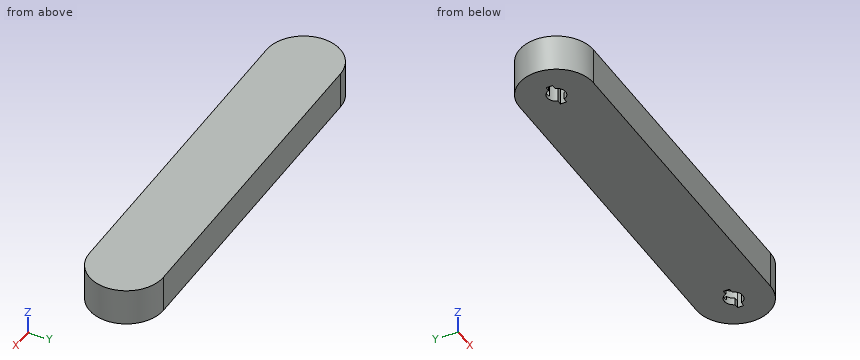
from build123d import *

# Parameters (mm, degrees)
BOSS_EXTRUDE1_DEPTH = 12.7
CUT_EXTRUDE1_DEPTH  = 6.35
CUT_EXTRUDE4_START  = 3.81
CUT_EXTRUDE4_DEPTH  = 3.81
CUT_EXTRUDE5_START  = 5.08
CUT_EXTRUDE5_DEPTH  = 5.08


with BuildPart() as part:
    # Sketch1 → Boss-Extrude1 (new body)
    with BuildSketch(Plane.XY):
        with BuildLine():
            Line((0, 0), (114.3, 0))
            ThreePointArc((114.3, 0), (127, -12.7), (114.3, -25.4))
            Line((114.3, -25.4), (0, -25.4))
            ThreePointArc((0, -25.4), (-12.7, -12.7), (0, 0))
        make_face()
    extrude(amount=-BOSS_EXTRUDE1_DEPTH)

    # Sketch2 → Cut-Extrude1 (cut)
    with BuildSketch(Plane(origin=(0, 0, -12.7), x_dir=(-1, 0, 0), z_dir=(0, 0, -1))):
        with BuildLine():
            Line((-118.872586333, -11.6205), (-118.872586333, -13.7795))
            Line((-118.872586333, -13.7795), (-117.285850758, -13.7795))
            ThreePointArc((-117.285850758, -13.7795), (-114.3, -15.875), (-111.314149242, -13.7795))
            Line((-111.314149242, -13.7795), (-109.727413667, -13.7795))
            Line((-109.727413667, -13.7795), (-109.727413667, -11.6205))
            Line((-109.727413667, -11.6205), (-111.314149242, -11.6205))
            ThreePointArc((-111.314149242, -11.6205), (-114.3, -9.525), (-117.285850758, -11.6205))
            Line((-117.285850758, -11.6205), (-118.872586333, -11.6205))
        make_face()
        with BuildLine():
            Line((-4.572586333, -11.6205), (-2.985850758, -11.6205))
            ThreePointArc((-2.985850758, -11.6205), (0, -9.525), (2.985850758, -11.6205))
            Line((2.985850758, -11.6205), (4.572586333, -11.6205))
            Line((4.572586333, -11.6205), (4.572586333, -13.7795))
            Line((4.572586333, -13.7795), (2.985850758, -13.7795))
            ThreePointArc((2.985850758, -13.7795), (0, -15.875), (-2.985850758, -13.7795))
            Line((-2.985850758, -13.7795), (-4.572586333, -13.7795))
            Line((-4.572586333, -13.7795), (-4.572586333, -11.6205))
        make_face()
    extrude(amount=-CUT_EXTRUDE1_DEPTH, mode=Mode.SUBTRACT)

    # Sketch3 → Cut-Extrude4 (cut)
    with BuildSketch(Plane(origin=(0, 0, -6.35), x_dir=(-1, 0, 0), z_dir=(0, 0, -1)).offset(CUT_EXTRUDE4_START)):
        with BuildLine():
            ThreePointArc((-113.2205, -8.127413667), (-116.769985033, -8.703371426), (-118.872586333, -11.6205))
            Line((-118.872586333, -11.6205), (-117.285850758, -11.6205))
            ThreePointArc((-117.285850758, -11.6205), (-115.647993548, -9.825362911), (-113.2205, -9.714149242))
            Line((-113.2205, -9.714149242), (-113.2205, -8.127413667))
        make_face()
        with BuildLine():
            Line((-109.727413667, -13.7795), (-111.314149242, -13.7795))
            ThreePointArc((-111.314149242, -13.7795), (-112.952006452, -15.574637089), (-115.3795, -15.685850758))
            Line((-115.3795, -15.685850758), (-115.3795, -17.272586333))
            ThreePointArc((-115.3795, -17.272586333), (-111.830014967, -16.696628574), (-109.727413667, -13.7795))
        make_face()
        with BuildLine():
            ThreePointArc((-1.0795, -8.127413667), (2.469985033, -8.703371426), (4.572586333, -11.6205))
            Line((4.572586333, -11.6205), (2.985850758, -11.6205))
            ThreePointArc((2.985850758, -11.6205), (1.347993548, -9.825362911), (-1.0795, -9.714149242))
            Line((-1.0795, -9.714149242), (-1.0795, -8.127413667))
        make_face()
        with BuildLine():
            ThreePointArc((1.0795, -17.272586333), (-2.469985033, -16.696628574), (-4.572586333, -13.7795))
            Line((-4.572586333, -13.7795), (-2.985850758, -13.7795))
            ThreePointArc((-2.985850758, -13.7795), (-1.347993548, -15.574637089), (1.0795, -15.685850758))
            Line((1.0795, -15.685850758), (1.0795, -17.272586333))
        make_face()
    extrude(amount=-CUT_EXTRUDE4_DEPTH, mode=Mode.SUBTRACT)

    # Sketch4 → Cut-Extrude5 (cut)
    with BuildSketch(Plane(origin=(0, 0, -6.35), x_dir=(-1, 0, 0), z_dir=(0, 0, -1)).offset(CUT_EXTRUDE5_START)):
        with BuildLine():
            Line((-113.2205, -9.714149242), (-113.2205, -8.127413667))
            Line((-113.2205, -8.127413667), (-115.3795, -8.127413667))
            Line((-115.3795, -8.127413667), (-115.3795, -9.714149242))
            ThreePointArc((-115.3795, -9.714149242), (-115.099019405, -9.627184843), (-114.8117038, -9.566506068))
            ThreePointArc((-114.8117038, -9.566506068), (-114.006661019, -9.538579869), (-113.2205, -9.714149242))
        make_face()
        with BuildLine():
            ThreePointArc((-115.3795, -15.685850758), (-114.3, -15.875), (-113.2205, -15.685850758))
            Line((-113.2205, -15.685850758), (-113.2205, -17.272586333))
            Line((-113.2205, -17.272586333), (-115.3795, -17.272586333))
            Line((-115.3795, -17.272586333), (-115.3795, -15.685850758))
        make_face()
    cut_extrude5 = extrude(amount=-CUT_EXTRUDE5_DEPTH, mode=Mode.SUBTRACT)

    # Mirror2: Cut-Extrude5 across plane
    add(cut_extrude5.mirror(Plane(origin=(57.15, 0, 0), x_dir=(0, 0, 1), z_dir=(1, 0, 0))), mode=Mode.SUBTRACT)


solid = part.part
Check sheet for the modelled part. Datum: model origin and axes. Units: mm. Coordinates: 2 decimals unless noted, no trailing zeros. Write each loop counter-clockwise with the first axis right and the second up, starting at its lowest first coordinate (ties: lowest second). Pieces come first, ordered by that corner, then holes.
Item 1: Cross-section at B-B on z = -1.75. Record the boundary of the cut face in (x, y).
Numbers:
outline: (0, -25.4) - (114.3, -25.4) arc R12.7 ccw to (114.3, 0) - (0, 0) arc R12.7 ccw to start
Item 2: Scan lines: probe 1 along X at (y, z) = (-14.5, -11); probe 2 along X at (y, z) = (-8.5, -7); probe 3 along X at (y, z) = (-19, -1.5). Record each from-to range of solid material in increasing order.
Numbers:
probe 1: x = -12.57 to -2.62, 2.62 to 111.68, 116.92 to 126.87
probe 2: x = -11.99 to -2.11, 1.08 to 113.22, 116.41 to 126.29
probe 3: x = -11.03 to 125.33
Item 3: Cross-section at A-A on z = -9. Count the separate pieces of the cut face and the enclosed holes in it, then the cut area to 3 significant figures.
Numbers:
separate pieces: 1
enclosed holes: 2
area: 3,300 mm2
Item 4: Cross-section at C-C on y = -3. Record the boundary of the cut face in (x, z), then the cut area to 3 significant figures.
Numbers:
outline: (-8.2, -12.7) - (122.5, -12.7) - (122.5, 0) - (-8.2, 0) - close
area: 1,660 mm2
Item 5: Depth check by flat-ended pin: pin 1 Ø0.6 at (y, z) = (-9, -11) entering from +X; pin 2 Ø0.8 at (x, y) = (0, -16.5) entering from +Z; pin 3 Ø4 at (y, z) = (-7, -10.5) entering from +X; pin 4 Ø1.4 at (y, z) = (-16.5, -11) entering from -X. Enter the tip coordinate at first touch or a pass-through.
Numbers:
pin 1: stops at x = 126.54
pin 2: stops at z = 0
pin 3: stops at x = 126.45
pin 4: stops at x = -12.32
